Geometry: final body of the model. Coordinates: model frame, mm. Coordinates: 2 decimals unless noted, no trailing zeros. Loops run counter-clockwise (first coordinate to the right, second up) from the corner with the lowest first, then second, coordinate; pieces in that order, holes last. Notation, with made-up numbers: (-3, 72.5) - (56, 72.5) arc R22 cw to (56, 98.5) - close; hole circle Ø2 at (6.25, -12). An arc over 180 degrees is marked (long way). Return JSON: item names as keys, results as strings.
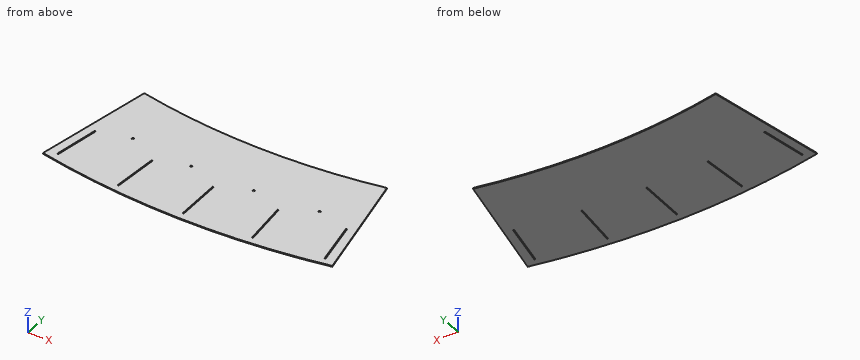
from build123d import *

# Parameters (mm, degrees)
SKETCH1_W           = 3.5
SKETCH1_H           = 150
BOSS_EXTRUDE1_DEPTH = 3
SKETCH3_R           = 4
CUT_EXTRUDE1_DEPTH  = 2


with BuildPart() as part:
    # Sketch1 → Boss-Extrude1 (new body)
    with BuildSketch(Plane.XY):
        with BuildLine():
            Line((-480.312372804, -2414.693360353), (-402.861514963, -2025.321604033))
            ThreePointArc((-402.861514963, -2025.321604033), (0, -2065), (402.861514963, -2025.321604033))
            Line((402.861514963, -2025.321604033), (480.312372804, -2414.693360353))
            ThreePointArc((480.312372804, -2414.693360353), (0, -2462), (-480.312372804, -2414.693360353))
        make_face()
        Polygon((-207.52154326, -2277.565997196), (-221.246786059, -2426.936736332), (-224.732103306, -2426.616480667), (-211.006860506, -2277.245741531), align=None, mode=Mode.SUBTRACT)
        with Locations((0, -2362)):
            Rectangle(SKETCH1_W, SKETCH1_H, mode=Mode.SUBTRACT)
        Polygon((-415.051950712, -2249.022885768), (-442.387279536, -2396.511121903), (-445.828671713, -2395.873297564), (-418.493342889, -2248.385061429), align=None, mode=Mode.SUBTRACT)
        Polygon((211.006860506, -2277.245741531), (224.732103306, -2426.616480667), (221.246786059, -2426.936736332), (207.52154326, -2277.565997196), align=None, mode=Mode.SUBTRACT)
        Polygon((418.493342889, -2248.385061429), (445.828671713, -2395.873297564), (442.387279536, -2396.511121903), (415.051950712, -2249.022885768), align=None, mode=Mode.SUBTRACT)
    extrude(amount=BOSS_EXTRUDE1_DEPTH)

    # Sketch3 → Cut-Extrude1 (cut)
    with BuildSketch(Plane.XY.offset(3)):
        with Locations((310.304616094, -2222)):
            Circle(SKETCH3_R)
        with Locations((103.730524899, -2241.163299042)):
            Circle(SKETCH3_R)
        with Locations((-103.730524899, -2241.163299042)):
            Circle(SKETCH3_R)
        with Locations((-310.304616094, -2222)):
            Circle(SKETCH3_R)
    extrude(amount=-CUT_EXTRUDE1_DEPTH, mode=Mode.SUBTRACT)


solid = part.part
Item 1: Section query B-B, the plane x = 377.5. Return loops of the section in (y, z), and give its area (3 significant figures).
Worked out:
{"outline": "(-2432.89, 0) - (-2030.2, 0) - (-2030.2, 3) - (-2432.89, 3) - close", "area": "1,210 mm^2"}
Item 2: Ray query, probe 1 along X at (y, z) = (-2222, 2); probe 2 along X at (y, z) = (-2272, 2.85); probe 3 along X at (y, z) = (-2406.5, 2.9). Return the intervals inside material, ascending. Write a range as from..to.
Worked out:
{"probe 1": "-441.98..-314.3, -306.3..306.3, 314.3..441.98", "probe 2": "-451.93..-422.87, -419.31..419.31, 422.87..451.93", "probe 3": "-478.68..-222.88, -219.37..-1.75, 1.75..219.37, 222.88..478.68"}
Item 3: Section query C-C, the plane y = -2137. Return loops of the section in (x, z), and give its area (3 significant figures).
Worked out:
{"outline": "(-425.08, 0) - (425.08, 0) - (425.08, 3) - (-425.08, 3) - close", "area": "2,550 mm^2"}
Item 4: Section query A-A, the plane z = 1.8. Count the separate pieces of the cut face and the enclosed holes in it, and give its area (3 significant figures).
Worked out:
{"separate pieces": "1", "enclosed holes": "9", "area": "350,000 mm^2"}
Item 5: First-contact query: pin 1 Ø0.9 at (y, z) = (-2377, 1.5) entering from -X; pin 2 Ø0.9 at (y, z) = (-2374, 1) entering from +X; pin 3 Ø7 at (x, y) = (-103.73, -2241.16) entering from +Z. Flat tips, straight axial feed; report the tip coordinate or a pass-through.
Worked out:
{"pin 1": "x = -472.9", "pin 2": "x = 472.31", "pin 3": "z = 1"}
